CAD build for the part. Positions are in the model's coordinates, mm. A direction names the side the tool comes from. Coordinates: 2 decimals unless noted, no trailing zeros. Loops run counter-clockwise (first coordinate to the right, second up) from the corner with the lowest first, then second, coordinate; pieces in that order, holes last. Notation, with made-up numbers: (21, -36.75) -> (52, -36.75) arc R21 ccw to (52, -23.75) -> close; hole circle Ø7 at (2, 78). An arc over 180 degrees is marked (long way). Write each question's results on one line, items separated by ' | '.
from build123d import *

# Parameters (mm, degrees)
F0_R     = 2
F1_DEPTH = 10
F0_R_2   = 2.1
F2_DEPTH = 2.6
F4_R     = 1
F5_W     = 2.1
F5_H     = 1


with BuildPart() as f1:
    # F0 (on Top) → F1 (new body)
    with BuildSketch(Plane.XY):
        with Locations((25, 0)):
            Circle(F0_R)
    extrude(amount=F1_DEPTH)

    # F0 (on Top) → F2 (join)
    with BuildSketch(Plane.XY):
        with BuildLine():
            Line((25, 7.5), (-25, 7.5))
            ThreePointArc((-25, 7.5), (-32.5, 0), (-25, -7.5))
            Line((-25, -7.5), (25, -7.5))
            ThreePointArc((25, -7.5), (32.5, 0), (25, 7.5))
        make_face()
        with Locations((-25, 0)):
            Circle(F0_R_2, mode=Mode.SUBTRACT)
        with Locations((25, 0)):
            Circle(F0_R, mode=Mode.SUBTRACT)
    extrude(amount=F2_DEPTH)

    # F4
    f4_edges = [f1.edges().sort_by_distance(p)[0] for p in [
        (23, 0, 10),
    ]]
    fillet(f4_edges, radius=F4_R)

    # F5 (on offset) → F6 (revolve)
    with BuildSketch(Plane.YZ.offset(25)):
        with Locations((-1.05, 7.6208)):
            Rectangle(F5_W, F5_H)
    revolve(axis=Axis((25, 0, 7.6208), (0, 0, -1)))


solid = f1.part
1) Pin check, flat tips, straight feed: pin 1 (5.5 mm diameter, centred on x = -25, y = 0, fed in from -Z); pin 2 (4 mm diameter, centred on x = 13, y = 4.5, fed in from +Z); pin 3 (1.5 mm diameter, centred on y = -2.5, z = 2.5, fed in from +X). Stop position of each tip, or through.
Outcome:
pin 1: stops at z = 0 | pin 2: stops at z = 2.6 | pin 3: stops at x = 32.29
2) Drill centre lines: L1, parallel to Y at x = -25, z = 2; L2, parallel to Z at x = 26.5, y = -5; L3, parallel to X at y = 0, z = 4.75. Where is each one in solid material? Low to high. Write a range as from..to.
Outcome:
L1: y = -7.5..-2.1, 2.1..7.5 | L2: z = 0..2.6 | L3: x = 23..27
3) Two-plate mould, pull along X, no slides. Class faces 4 (the cylindrical face through (-32.5, 0.16, 1.28)), 5 (the cylindrical face through (-22.997, 0.631, 1.282)), 6 (the flat face through (25, 0, 10)): pulls with the +X half, pulls with the -X half, needs draft (parallel to the pull), parting line crosses it, or undercut.
Outcome:
face 4: pulls with the -X half | face 5: undercut | face 6: needs draft
4) Slice it at A-A (x = 9.5). Write the cut outline in (y, z).
Outcome:
outline: (-7.5, 0) -> (7.5, 0) -> (7.5, 2.6) -> (-7.5, 2.6) -> close
5) Which spindle directions (+Z, -Z, +X, -X, +Y, -Y) get a long thin tool onto all of the face, cutting with end or side? Do faces 1 (the cylindrical face through (23, 0, 5)), 2 (the cylindrical face through (23.23, -1.13, 7.63)), 3 (the flat face through (0, 7.5, 1)). Say none if no direction does.
Outcome:
face 1: none | face 2: +Z | face 3: +Z, -Z, +X, -X, +Y
6) Slice it at C-C (y = 6.25). Write the cut outline in (x, z).
Outcome:
outline: (-29.15, 0) -> (29.15, 0) -> (29.15, 2.6) -> (-29.15, 2.6) -> close
7) Slice it at B-B (z = 5.75). Write the cut outline in (x, y).
Outcome:
outline: circle Ø4 at (25, 0)
